Autodesk Inventor part; units mm, degrees
ref_plane "Plano inicial" through (0, 0, 0) normal (0, 0, 1) x (1, 0, 0)
ref_plane "Plano final" through (0, 0, 550) normal (0, 0, 1) x (1, 0, 0)
ref_plane "YZ Plane" through (0, 0, 0) normal (1, 0, 0) x (0, 1, 0)
ref_plane "Plano inicial" through (0, 0, 0) normal (0, 0, 1) x (1, 0, 0)
ref_plane "Plano final" through (0, 0, 550) normal (0, 0, 1) x (1, 0, 0)
sketch "Rascunho" plane through (0, 0, 0) normal (0, 0, 1) x (1, 0, 0)
  line L0 (-15, -8.4) -> (-15, 8.4)
  line L1 (-8.4, 15) -> (8.4, 15)
  line L2 (15, 8.4) -> (15, -8.4)
  line L3 (8.4, -15) -> (-8.4, -15)
  arc A0 (-15, -8.4) -> (-8.4, -15) centre (-8.4, -8.4) ccw
  arc A1 (-8.4, 15) -> (-15, 8.4) centre (-8.4, 8.4) ccw
  arc A2 (15, 8.4) -> (8.4, 15) centre (8.4, 8.4) ccw
  arc A3 (8.4, -15) -> (15, -8.4) centre (8.4, -8.4) ccw
  arc A4 (-8.4, 12) -> (-12, 8.4) centre (-8.4, 8.4) ccw
  line L4 (-8.4, 12) -> (8.4, 12)
  arc A5 (12, 8.4) -> (8.4, 12) centre (8.4, 8.4) ccw
  line L5 (12, 8.4) -> (12, -8.4)
  arc A6 (8.4, -12) -> (12, -8.4) centre (8.4, -8.4) ccw
  line L6 (8.4, -12) -> (-8.4, -12)
  arc A7 (-12, -8.4) -> (-8.4, -12) centre (-8.4, -8.4) ccw
  line L7 (-12, -8.4) -> (-12, 8.4)
  line L8 (0, 22.9137) -> (0, -22.9137) construction
  line L9 (-22.9137, 0) -> (22.9137, 0) construction
  dimension "d7" = 6.6
  dimension "d10" = 30
  dimension "d11" = 30
  dimension "d12" = 3
  dimension "d15" = 15
  dimension "d16" = 15
extrude "Corpo" add sketch "Rascunho" along normal blind 200 from surface at 0
sketch "Sketch3" plane through (0, 0, 0) normal (0, 0, 1) x (1, 0, 0)
  line L0 (0, 0) -> (10, 0)
ref_plane "Work Plane3" through (0, 0, 0) normal (0, -1, 0) x (1, 0, 0)
sketch "Sketch4" plane through (0, 0, 0) normal (0, -1, 0) x (1, 0, 0)
  line L0 (-2, 0) -> (12, 0)
  line L1 (-2, 550) -> (12, 550)
  dimension "d18" = 550
equation "\"d7\" = G_IR"
equation "\"d10\" = G_H"
equation "\"d11\" = G_W"
equation "\"d12\" = G_T"
equation "\"d15\" = 0.5 * d10"
equation "\"d16\" = 0.5 * d11"
equation "\"G_W\" = 30"
equation "\"G_H\" = 30"
equation "\"G_T\" = 3"
equation "\"G_IR\" = 6.6"
equation "\"G_L\" = d18"
equation "\"G_OFFSET_START\" = 0"
equation "\"G_OFFSET_END\" = 0"
properties part number "tubo extensão menor" material "Aço, suave"
Work out the finished part from the listing and answer in its coordinate system (mm). A direction names the side the tool comes from. Give positions to 0.01 mm unless a question says otherwise; leave off trailing zeros. Write each loop counter-clockwise with the first axis right and the second up, starting at its lowest first coordinate (ties: lowest second). Pieces come first, ordered by that corner, then holes. Notation, with made-up numbers: (14.25, 9.5) - (32.25, 9.5) arc R21 ccw to (32.25, 45.5) - close; hole circle Ø11 at (-2.5, 62.25). An arc over 180 degrees is marked (long way). Use one line per item in the form item = value.
1. Consider L1, parallel to X at y = -1.25, z = 183; L2, parallel to X at y = -9, z = 148. Determine where each line is inside the solid, lowest interval first.
Filled in:
L1 = -15 to -12, 12 to 15
L2 = -14.97 to -11.95, 11.95 to 14.97
2. Determine the mould class of faces 1 (the face through (12.2, -1, 200)), 2 (the face through (-12, 0, 99)), 3 (the face through (-13.118, 13.015, 98.6)) for opening direction Y: released by +Y, released by -Y, zero draft, split by the parting line, or undercut.
Filled in:
face_1 = zero draft
face_2 = undercut
face_3 = released by +Y
3. A cutting plane is placed at C-C (z = 169). Write down the section's boundary in (x, y), and give its area (3 significant figures).
Filled in:
outline = (-15, -8.4) arc R6.6 ccw to (-8.4, -15) - (8.4, -15) arc R6.6 ccw to (15, -8.4) - (15, 8.4) arc R6.6 ccw to (8.4, 15) - (-8.4, 15) arc R6.6 ccw to (-15, 8.4) - close; hole (-12, -8.4) arc R3.6 ccw to (-8.4, -12) - (8.4, -12) arc R3.6 ccw to (12, -8.4) - (12, 8.4) arc R3.6 ccw to (8.4, 12) - (-8.4, 12) arc R3.6 ccw to (-12, 8.4) - close
area = 298 mm^2
4. A cutting plane is placed at A-A (x = 4.25). Write down the section's boundary in (y, z), and give its area (3 significant figures).
Filled in:
outline = (-15, 0) - (-12, 0) - (-12, 200) - (-15, 200) - close; (12, 0) - (15, 0) - (15, 200) - (12, 200) - close
area = 1,200 mm^2
5. For faces 4 (the face through (-15, 0, 99)), 5 (the face through (10.97, -10.92, 98.6)), determine the directions among +Z, -Z, +X, -X, +Y, -Y from which every point of the face is accessible in a straight line to the end or side of a thin tool.
Filled in:
face_4 = +Z, -Z, -X, +Y, -Y
face_5 = +Z, -Z
